from build123d import *

# Parameters (mm, degrees)
BOSS_EXTRU_1_DEPTH      = 3
BOSS_EXTRU_2_DEPTH      = 20
BOSS_EXTRU_3_DEPTH      = 3
ENL_V_MAT_EXTRU_2_DEPTH = 10
ESQUISSE9_R             = 1.775
ESQUISSE9_W             = 2.5
ESQUISSE9_H             = 16
ENL_V_MAT_EXTRU_3_DEPTH = 10
CONG_1_R                = 10
CONG_2_R                = 10


with BuildPart() as part:
    # Esquisse1 → Boss.-Extru.1 (new body)
    with BuildSketch(Plane.XY):
        with BuildLine():
            Line((0, 0), (10, 0))
            ThreePointArc((10, 0), (48.5, 38.5), (87, 0))
            Line((87, 0), (97, 0))
            Line((97, 0), (97, -3))
            Line((97, -3), (0, -3))
            Line((0, -3), (0, 0))
        make_face()
    extrude(amount=BOSS_EXTRU_1_DEPTH)

    # Esquisse2 → Boss.-Extru.2 (add)
    with BuildSketch(Plane.XY.offset(3)):
        Polygon((10, 0), (0, 0), (0, -3), (14, -3), (14, 0), align=None)
        with BuildLine():
            ThreePointArc((87, 0), (48.5, 38.5), (10, 0))
            Line((10, 0), (14, 0))
            ThreePointArc((14, 0), (48.5, 34.5), (83, 0))
            Line((83, 0), (87, 0))
        make_face()
        Polygon((97, 0), (87, 0), (83, 0), (83, -3), (97, -3), align=None)
    extrude(amount=BOSS_EXTRU_2_DEPTH)

    # Esquisse4 → Boss.-Extru.3 (add)
    with BuildSketch(Plane(origin=(0, 0, 0), x_dir=(-1, 0, 0), z_dir=(0, 0, -1))):
        with BuildLine():
            Line((-64.5, -3), (-32.5, -3))
            ThreePointArc((-32.5, -3), (-48.5, -19), (-64.5, -3))
        make_face()
    extrude(amount=-BOSS_EXTRU_3_DEPTH)

    # Esquisse7 → Enl_v. mat.-Extru.2 (cut)
    with BuildSketch(Plane(origin=(0, 0, 0), x_dir=(1, 0, 0), z_dir=(0, 1, 0))):
        with BuildLine():
            Line((3.5, -18), (3.5, -12))
            ThreePointArc((3.5, -12), (5, -10.5), (6.5, -12))
            Line((6.5, -12), (6.5, -18))
            ThreePointArc((6.5, -18), (5, -19.5), (3.5, -18))
        make_face()
        with BuildLine():
            Line((90.5, -18), (90.5, -12))
            ThreePointArc((90.5, -12), (92, -10.5), (93.5, -12))
            Line((93.5, -12), (93.5, -18))
            ThreePointArc((93.5, -18), (92, -19.5), (90.5, -18))
        make_face()
    extrude(amount=-ENL_V_MAT_EXTRU_2_DEPTH, mode=Mode.SUBTRACT)

    # Esquisse9 → Enl_v. mat.-Extru.3 (cut)
    with BuildSketch(Plane.XY.offset(3)):
        with Locations((40.39013432, 6.64)):
            Circle(ESQUISSE9_R)
        with Locations((56.39013432, 6.64)):
            Circle(ESQUISSE9_R)
        with Locations((40.39013432, -9.36)):
            Circle(ESQUISSE9_R)
        with Locations((56.39013432, -9.36)):
            Circle(ESQUISSE9_R)
        with Locations((41.64013432, -1.36)):
            Rectangle(ESQUISSE9_W, ESQUISSE9_H)
        with Locations((55.14013432, -1.36)):
            Rectangle(ESQUISSE9_W, ESQUISSE9_H)
    extrude(amount=-ENL_V_MAT_EXTRU_3_DEPTH, mode=Mode.SUBTRACT)

    # Cong_1
    cong_1_edges = [part.edges().sort_by_distance(p)[0] for p in [
        (97, -1.5, 0),
    ]]
    fillet(cong_1_edges, radius=CONG_1_R)

    # Cong_2
    cong_2_edges = [part.edges().sort_by_distance(p)[0] for p in [
        (0, -1.5, 0),
    ]]
    fillet(cong_2_edges, radius=CONG_2_R)


solid = part.part
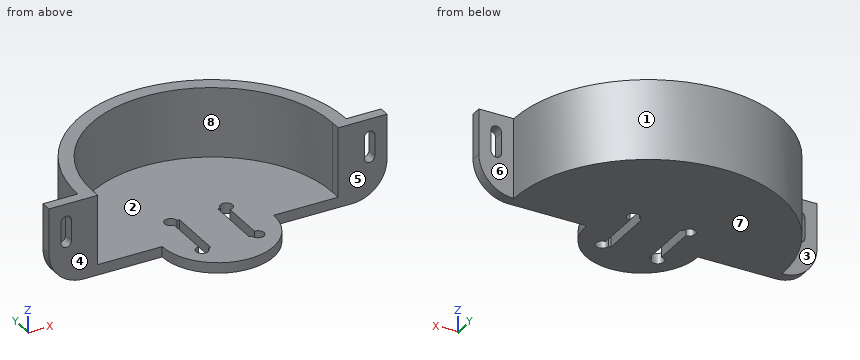
Can you work these out from the model? Positions are in its coordinate system, mm. Face numbers are marked on the shaded views. A direction names the side the tool comes from. Give positions to 0.01 mm unless a question says otherwise; leave off trailing zeros. Order: outer loops, then holes, each group sorted by start corner. A loop starts at its lowest first (then second) coordinate and runs counter-clockwise, first axis right, second up. Notation, with made-up numbers: M 46.5,1 L 67.5,1 A6 ccw 67.5,9 Z; hole C 80.25,75.5 d7. An arc over 180 degrees is marked long. Use a Markdown table: item, result. Add a question column.
Item 1: Will these pins go through, and if not, where does the flat tip stop? pin 1 (2 mm diameter, centred on y = 28, z = 5.5, fed in from -X); pin 2 (4 mm diameter, centred on x = 72, z = 8, fed in from -Y); pin 3 (8 mm diameter, centred on x = 61.5, z = 17.5, fed in from +Y); pin 4 (4 mm diameter, centred on x = 40.39, y = 6.64, fed in from -Z).
Item 2: We'd pull the mould along X, two halves only. Please class the marked faces 1, 2 and 3: +X half, -X half, draft (parallel to the pull), parting line (faces both ways), or undercut.
Item 3: For the marked faces 4, 5, 6, 7 and 8, which set-ups out of +Z, -Z, +X, -X, +Y, -Y let a thin tool reach every point of the face, with its end or its side?
Item 4: Suppose I cut it at C-C (x = 48.5). List the corners of the cut face in (y, z) for me.
Item 5: If I drill on L1, parallel to Z at x = 42, y = -14; L2, parallel to X at y = 7, z = 15.75; L3, parallel to Y at x = 92, z = 1.75, over which ranges is the centre line in solid material (lowest first)? Write a range as [from, to].
Item 6: Suppose I cut it at B-B (z = 21). List the corners of the cut face in (x, y) for me.
Item 7: Suppose I cut it at D-D (y = 25.5). List the corners of the cut face in (x, z) for me, then the cut area to 3 significant figures.
Item 8: Suppose I cut it at A-A (y = -4). List the corners of the cut face in (x, z) for me, then the cut area to 3 significant figures.
Answer sheet:
| question | item | result |
|---|---|---|
| 1 | pin 1 | stops at x = 21.05 |
| 1 | pin 2 | stops at y = 23.24 |
| 1 | pin 3 | stops at y = 37.43 |
| 1 | pin 4 | stops at z = 0 |
| 2 | face 1 | parting line |
| 2 | face 2 | undercut |
| 2 | face 3 | draft |
| 3 | face 4 | +Z, -Z, -X, -Y |
| 3 | face 5 | +Z, -Z, +X, -Y |
| 3 | face 6 | +Z, -Z, +X, +Y |
| 3 | face 7 | -Z, +X, -X, +Y, -Y |
| 3 | face 8 | +Z, -Y |
| 4 | outline | M -19,0 L 38.5,0 L 38.5,23 L 34.5,23 L 34.5,3 L -19,3 Z |
| 5 | L1 | z = [0, 3] |
| 5 | L2 | x = [10.64, 14.72], [82.28, 86.36] |
| 5 | L3 | y = [-3, 0] |
| 6 | outline | M 0,-3 L 14,-3 L 14,0 A34.5 cw 83,0 L 83,-3 L 97,-3 L 97,0 L 87,0 A38.5 ccw 10,0 L 0,0 Z |
| 7 | outline | M 19.66,0 L 77.34,0 L 77.34,23 L 71.74,23 L 71.74,3 L 25.26,3 L 25.26,23 L 19.66,23 Z |
| 7 | area | 397 mm² |
| 8 | outline | M 32.53,0 L 40.39,0 L 40.39,3 L 32.53,3 Z; M 42.89,0 L 53.89,0 L 53.89,3 L 42.89,3 Z; M 56.39,0 L 64.47,0 L 64.47,3 L 56.39,3 Z |
| 8 | area | 80.8 mm² |
